Autodesk Inventor part; units mm, degrees
ref_plane "Work Plane1" through (-205, 2, 0) normal (0, 1, 0) x (1, 0, 0)
ref_plane "YZ Plane" through (0, 0, 0) normal (1, 0, 0) x (0, 1, 0)
ref_plane "XZ Plane" through (0, 0, 0) normal (0, 1, 0) x (-1, 0, 0)
ref_plane "Work Plane1" through (-205, 2, 0) normal (0, 1, 0) x (1, 0, 0)
sketch "Sketch2" plane through (-205, 2, 0) normal (0, 1, 0) x (1, 0, 0)
  circle A0 centre (86.5, -146.525) radius 1.675
  circle A1 centre (86.5, -146.525) radius 1.675
  circle A2 centre (86.5, -146.525) radius 4.5
  circle A3 centre (172.5, -35.525) radius 1.675
  circle A4 centre (172.5, -35.525) radius 1.675
  circle A5 centre (172.5, -35.525) radius 4.5
  circle A6 centre (132.5, -283.785) radius 1.675
  circle A7 centre (132.5, -283.785) radius 6.215
  line L0 (0, -290) -> (155, -290)
  circle A8 centre (7.5, -283.785) radius 1.675
  circle A9 centre (7.5, -283.785) radius 4.5
  circle A10 centre (7.5, -167.775) radius 1.675
  circle A11 centre (7.5, -167.775) radius 4.5
  circle A12 centre (7.5, -17.325) radius 1.675
  circle A13 centre (7.5, -17.325) radius 4.5
  line L1 (0, -290) -> (132.5, -290)
  line L2 (91, -146.525) -> (138.3655, -281.7302)
  line L3 (91, -146.525) -> (176.0383, -38.3054)
  line L4 (172.5, -31.025) -> (7.9941, -12.8522)
  line L5 (7.9941, -12.8522) -> (0, -12.8522)
  line L6 (0, -12.8522) -> (0, -290)
  point P0 (205, 0)
  dimension "d3" = 9
  dimension "d7" = 9
  dimension "d4" = 9
  dimension "d5" = 9
  dimension "d6" = 9
extrude "Extrusion1" add sketch "Sketch2" along normal blind 0.2 contours A2 | L2 A7 L0 L6 L5 A13 L4 A5 L3 | A7 | A5 | A13 L5 | A9 | A11 picked at (10.9979, -16.8298)
properties part number "base_main_pcb_full_itr3"
Verification items for the finished model (mm, model axes). Give positions to 0.01 mm unless a question says otherwise; leave off trailing zeros. Write each loop counter-clockwise with the first axis right and the second up, starting at its lowest first coordinate (ties: lowest second). Pieces come first, ordered by that corner, then holes. Notation, with made-up numbers: M 67,29 L 107,29 A22 ccw 107,46 Z; hole C 36,40 d8. An arc over 180 degrees is marked long. Use CSV: the item, a comma, the result in double quotes.
1) Go/stop test with a flat-tipped pin: pin 1 Ø2 at (x, z) = (-197.5, 283.785) entering from -Y. Record where the tip stops, or that it passes through.
Final values:
pin 1,"through"
2) Cross-section at B-B (y = 2.15). State how many separate pieces and enclosed holes the cut face has, plus the area to 3 significant figures.
Final values:
separate pieces,"1"
enclosed holes,"6"
area,"34,000 mm²"
3) Cross-section at C-C (x = -145.5). Enter the section's corners in (y, z), plus the area to 3 significant figures.
Final values:
outline,"M 2,18.54 L 2.2,18.54 L 2.2,290 L 2,290 Z"
area,"54.3 mm²"
4) Cross-section at D-D (z = 151). Enter the section's corners in (x, y).
Final values:
outline,"M -205,2 L -112.43,2 L -112.43,2.2 L -205,2.2 Z"
5) Cross-section at A-A (x = -100). Enter the section's corners in (y, z), plus the area to 3 significant figures.
Final values:
outline,"M 2,23.57 L 2.2,23.57 L 2.2,128.71 L 2,128.71 Z; M 2,186.49 L 2.2,186.49 L 2.2,290 L 2,290 Z"
area,"41.7 mm²"
6) Material ranges on line 1 along Z through (x, y) = (-197.5, 2.1); line 2 along Z through (x, y) = (-118.5, 2.15); line 3 along X through (y, z) = (2.15, 37), recorded low to high.
Final values:
line 1,"12.85 to 15.65, 19 to 166.1, 169.45 to 282.11, 285.46 to 290"
line 2,"21.52 to 144.85, 148.2 to 290"
line 3,"-205 to -33.29, -31.71 to -28.25"
